Here's how the part is built. I have some questions about the finished solid (model axes, mm). Face numbers are marked on the shaded views. Round coordinates to 2 decimals unless told otherwise and drop trailing zeros. Write each loop counter-clockwise with the first axis right and the second up, starting at its lowest first coordinate (ties: lowest second). Pieces come first, ordered by that corner, then holes. Notation, with made-up numbers: M 44.5,18.25 L 77.5,18.25 A35 cw 77.5,57.25 Z; hole C 73.25,74.25 d3. An arc over 180 degrees is marked long. Write item = value, one per line. Start each with the question number.
(1) I want a section at D-D (x = 54). List the corners of the cut face in (y, z) for me.
(2) I want a section at A-A (z = -33). List the corners of the cut face in (x, y) for me.
(3) I need wall thicknesses on line 1 along X through (y, z) = (4, -66); line 2 along Y through (x, z) = (2.2, -33); line 3 along X through (y, z) = (7.5, -65). Which ranges of each line are inside material? Lowest first, please.
(4) If we mould it in two halves opening along Z, with no side actions, what happens to the marked faces 1, 2, 3 and 4? For each: released by +Z, released by -Z, zero draft, split by the parting line, or undercut.
(5) Will these pins go through, and if not, where does the flat tip stop? pin 1 Ø1 at (y, z) = (21, -61.5) entering from +X; pin 2 Ø0.6 at (x, y) = (50, 12.5) entering from +Z; pin 3 Ø0.8 at (x, z) = (78, -77.5) entering from +Y.
(6) I want a section at C-C (y = 5.5). Give the number of separate pieces and of enclosed holes in the cut face, and give its area (3 significant figures).
(7) I want a section at B-B (z = -54). List the corners of the cut face in (x, y) for me, and give its area (3 significant figures).
Autodesk Fusion 360 part; units mm, degrees
sketch "Sketch1" plane through (0, 0, 0) normal (0, 1, 0) x (1, 0, 0)
  line L0 (0, 0) -> (120, 0)
  line L1 (120, 0) -> (120, 85)
  line L2 (120, 85) -> (0, 85)
  line L3 (0, 85) -> (0, 0)
extrude "Extrude1" add sketch "Sketch1" along normal blind 3
sketch "Sketch2" plane through (0, 3, 0) normal (0, 1, 0) x (-1, 0, 0)
  line L0 (0, -85) -> (0, 0)
  line L1 (0, 0) -> (-120, 0)
  line L2 (-120, 0) -> (-120, -85)
  line L3 (-120, -85) -> (0, -85)
  line L4 (-60, -85) -> (-60, 0)
  line L5 (-60, -76.9514) -> (-120, -76.9514)
  line L6 (-77.8086, -80) -> (-77.8086, -73)
  circle A0 centre (-77.8086, -76.9514) radius 3.5
  circle A1 centre (-105.7039, -76.9514) radius 3.5
  dimension "d3" = 7
  dimension "d4" = 7
sketch "Sketch3" plane through (0, 3, 0) normal (0, 1, 0) x (-1, 0, 0)
  line L0 (-60, -10.9513) -> (-119.9962, -10.9513)
  line L1 (-60, -85) -> (-60, 0)
  line L2 (-60, -26.1629) -> (-72, -26.1629)
  line L3 (-62.566, -28.9848) -> (-62.566, -23)
  circle A0 centre (-62.566, -26.1629) radius 3.5
  line L4 (-107.0217, -24.9659) -> (-120.1868, -24.9659)
  line L5 (-110.7456, -28) -> (-110.7456, -22)
  circle A1 centre (-110.7456, -25) radius 2.5
  line L6 (-55, 0) -> (-55.9638, 0)
  line L7 (-55.9638, 0) -> (-55.9638, -85)
  line L8 (-55.9638, -85) -> (-55, -85)
  line L9 (-55, -85) -> (-55, 0)
  line L10 (0, 0) -> (-120, 0)
  line L11 (-120, -85) -> (0, -85)
  dimension "d5" = 7
  dimension "d6" = 5
extrude "Extrude2" add sketch "Sketch2" sketch "Sketch3" along normal blind 5 contours L5 A0 | L5 L6 A0 | L5 A1 | L5 A1 | L5 L6 A0 of sketch 2 contours L1 A0 | L1 L2 A0 | L1 L2 A0 | L4 L5 A1 | L4 L5 A1 | L4 L5 A1 | L4 L5 A1
hole "Hole1" at (77.8086, 8, -76.9514) direction (0, -1, 0) diameter 2.529 depth 4 tip angle 180
hole "Hole2" at (105.7039, 8, -76.9514) direction (0, -1, 0) diameter 2.529 depth 4 tip angle 180
hole "Hole3" at (62.566, 8, -26.1629) direction (0, -1, 0) diameter 2.529 depth 4 tip angle 180
hole "Hole4" at (110.7456, 8, -25) direction (0, -1, 0) diameter 2.529 depth 4 tip angle 180
sketch "Sketch4" plane through (0, 3, 0) normal (0, 1, 0) x (-1, 0, 0)
  circle A0 centre (-62.566, -26.1629) radius 3.5
  circle A1 centre (-105.7039, -76.9514) radius 3.5
  circle A2 centre (-77.8086, -76.9514) radius 3.5
  circle A3 centre (-110.7456, -25) radius 2.5
  line L0 (0, -85) -> (0, 0)
  line L1 (0, 0) -> (-120, 0)
  line L2 (-120, 0) -> (-120, -85)
  line L3 (-120, -85) -> (0, -85)
  line L4 (-50, -15) -> (-22, -15)
  line L5 (-22, -15) -> (-22, -70)
  line L6 (-22, -70) -> (-50, -70)
  line L7 (-50, -70) -> (-50, -15)
  line L8 (-22, -18) -> (-50, -18)
  circle A4 centre (-25, -18) radius 3
  circle A5 centre (-47, -18) radius 3
  line L9 (-20, -70) -> (-52, -70)
  line L10 (-52, -70) -> (-52, -69)
  line L11 (-52, -69) -> (-20, -69)
  line L12 (-20, -69) -> (-20, -70)
  dimension "d21" = 6
  dimension "d22" = 6
extrude "Extrude3" add sketch "Sketch4" along normal blind 5 contours L8 A5 | L8 A5 | L8 A4 | L5 L6 L7 L9 L11 | L7 L9 L10 L11 | L8 A4 | L5 L9 L11 L12
hole "Hole5" at (25, 8, -18) direction (0, -1, 0) diameter 2.529 depth 4 tip angle 180
hole "Hole6" at (47, 8, -18) direction (0, -1, 0) diameter 2.529 depth 4 tip angle 180
sketch "Sketch5" plane through (0, 3, 0) normal (0, 1, 0) x (-1, 0, 0)
  circle A0 centre (-47, -18) radius 3
  circle A1 centre (-25, -18) radius 3
  line L0 (-20, -69) -> (-20, -70)
  line L1 (-20, -70) -> (-52, -70)
  line L2 (-52, -70) -> (-52, -69)
  line L3 (-52, -69) -> (-20, -69)
  circle A2 centre (-62.566, -26.1629) radius 3.5
  circle A3 centre (-105.7039, -76.9514) radius 3.5
  circle A4 centre (-77.8086, -76.9514) radius 3.5
  circle A5 centre (-110.7456, -25) radius 2.5
  line L4 (0, -85) -> (0, 0)
  line L5 (0, 0) -> (-120, 0)
  line L6 (-120, 0) -> (-120, -85)
  line L7 (-120, -85) -> (0, -85)
  line L8 (-20, -70) -> (-52, -70)
  line L9 (-52, -70) -> (-52, -73)
  line L10 (-52, -73) -> (-20, -73)
  line L11 (-20, -73) -> (-20, -70)
extrude "Extrude4" add sketch "Sketch5" along normal blind 5 contours L1 L8 L9 L10 L11
sketch "Sketch6" plane through (0, 8, 0) normal (0, 1, 0) x (-1, 0, 0)
  line L0 (-20, -69) -> (-52, -69)
  line L1 (-52, -69) -> (-52, -73)
  line L2 (-52, -73) -> (-20, -73)
  line L3 (-20, -73) -> (-20, -69)
  line L4 (-20, -73) -> (-52, -73)
  line L5 (-52, -73) -> (-52, -71)
  line L6 (-52, -71) -> (-20, -71)
  line L7 (-20, -71) -> (-20, -73)
extrude "Extrude5" add sketch "Sketch6" along normal blind 5 contours L1 L2 L3 L4 L5 L6 L7
sketch "Sketch7" plane through (0, 0, -71) normal (0, 0, 1) x (1, 0, 0)
  line L0 (20, 8) -> (52, 8)
  line L1 (52, 8) -> (52, 13)
  line L2 (52, 13) -> (20, 13)
  line L3 (20, 13) -> (20, 8)
  line L4 (48.0761, 13) -> (52, 13)
  line L5 (52, 13) -> (52, 10.5)
  line L6 (52, 10.5) -> (48.0761, 10.5)
  line L7 (48.0761, 10.5) -> (48.0761, 13)
extrude "Extrude6" add sketch "Sketch7" along normal blind 4 contours L1 L2 L4 L5 L6 L7
sketch "Sketch8" plane through (52, 0, 0) normal (1, 0, 0) x (0, 0, -1)
  line L0 (69, 3) -> (73, 3)
  line L1 (73, 3) -> (73, 13)
  line L2 (73, 13) -> (67, 13)
  line L3 (67, 13) -> (67, 10.5)
  line L4 (67, 10.5) -> (71, 10.5)
  line L5 (71, 10.5) -> (71, 8)
  line L6 (71, 8) -> (69, 8)
  line L7 (69, 8) -> (69, 3)
  line L8 (67, 11.75) -> (71, 10.5)
extrude "Extrude7" cut sketch "Sketch8" against normal blind 4 contours L3 L4 L8
sketch "Sketch9" plane through (0, 3, 0) normal (0, 1, 0) x (-1, 0, 0)
  line L0 (-52, -73) -> (-52, -69)
  line L1 (-52, -69) -> (-20, -69)
  line L2 (-20, -69) -> (-20, -73)
  line L3 (-20, -73) -> (-52, -73)
  circle A0 centre (-47, -18) radius 3
  circle A1 centre (-25, -18) radius 3
  circle A2 centre (-62.566, -26.1629) radius 3.5
  circle A3 centre (-105.7039, -76.9514) radius 3.5
  circle A4 centre (-77.8086, -76.9514) radius 3.5
  circle A5 centre (-110.7456, -25) radius 2.5
  line L4 (0, -85) -> (0, 0)
  line L5 (0, 0) -> (-120, 0)
  line L6 (-120, 0) -> (-120, -85)
  line L7 (-120, -85) -> (0, -85)
  line L8 (0, 0) -> (-2.9371, 0)
  line L9 (-2.9371, 0) -> (-2.9371, -85)
  line L10 (-2.9371, -85) -> (0, -85)
  line L11 (0, -85) -> (0, 0)
  line L12 (0, 0) -> (-3, 0)
  line L13 (-3, 0) -> (-3, -85)
  line L14 (-3, -85) -> (0, -85)
  line L15 (0, -85) -> (0, 0)
  dimension "d39" = 3
extrude "Extrude8" add sketch "Sketch9" along normal blind 30 contours L4 L5 L7 L8 L9 L10 L11 L12 L14 L15
sketch "Sketch10" plane through (2.9371, 0, 0) normal (1, 0, 0) x (0, 0, -1)
  line L0 (0, 3) -> (85, 3)
  line L1 (85, 3) -> (85, 33)
  line L2 (85, 33) -> (0, 33)
  line L3 (0, 33) -> (0, 3)
  line L4 (0, 33) -> (3, 33)
  line L5 (3, 33) -> (3, 3)
  line L6 (3, 3) -> (0, 3)
  line L7 (0, 3) -> (0, 33)
  line L8 (85, 33) -> (82, 33)
  line L9 (82, 33) -> (82, 3)
  line L10 (82, 3) -> (85, 3)
  line L11 (85, 3) -> (85, 33)
  dimension "d42" = 3
  dimension "d43" = 3
extrude "Extrude9" add sketch "Sketch10" along normal blind 15 contours L0 L2 L3 L4 L5 L6 L7 | L0 L1 L2 L8 L9 L10 L11
sketch "Sketch11" plane through (0, 0, -3) normal (0, 0, -1) x (-1, 0, 0)
  line L0 (-2.9371, 3) -> (-2.9371, 33)
  line L1 (-2.9371, 33) -> (-17.9371, 33)
  line L2 (-17.9371, 33) -> (-17.9371, 3)
  line L3 (-17.9371, 3) -> (-2.9371, 3)
  line L4 (-2.9371, 33) -> (-17.9371, 3)
extrude "Extrude10" cut sketch "Sketch11" against normal blind 4 contours L1 L2 L4
sketch "Sketch13" plane through (0, 3, 0) normal (0, 1, 0) x (-1, 0, 0)
  line L0 (-17.9371, -82) -> (-2.9371, -82)
  line L1 (-2.9371, -82) -> (-2.9371, -3)
  line L2 (-2.9371, -3) -> (-17.9371, -3)
  line L3 (-17.9371, -3) -> (-17.9371, 0)
  line L4 (-17.9371, 0) -> (-120, 0)
  line L5 (-120, 0) -> (-120, -85)
  line L6 (-120, -85) -> (-17.9371, -85)
  line L7 (-52, -73) -> (-52, -69)
  line L8 (-52, -69) -> (-20, -69)
  line L9 (-20, -69) -> (-20, -73)
  line L10 (-20, -73) -> (-52, -73)
  circle A0 centre (-47, -18) radius 3
  circle A1 centre (-25, -18) radius 3
  circle A2 centre (-62.566, -26.1629) radius 3.5
  circle A3 centre (-105.7039, -76.9514) radius 3.5
  circle A4 centre (-77.8086, -76.9514) radius 3.5
  circle A5 centre (-110.7456, -25) radius 2.5
  line L11 (-14.9586, -82) -> (-17.7256, -82)
  line L12 (-17.7256, -82) -> (-17.7256, -39)
  line L13 (-17.7256, -39) -> (-14.9586, -39)
  line L14 (-14.9586, -39) -> (-14.9586, -82)
  line L15 (-17.9371, -85) -> (-17.9371, -82)
extrude "Extrude12" add sketch "Sketch13" along normal blind 25 contours L0 L11 L12 L13 L14
sketch "Sketch14" plane through (0, 0, -82) normal (0, 0, 1) x (1, 0, 0)
  line L0 (17.7256, 28) -> (17.7256, 3)
  line L1 (17.7256, 3) -> (17.9371, 3)
  line L2 (17.9371, 3) -> (17.9371, 33)
  line L3 (17.9371, 33) -> (2.9371, 33)
  line L4 (2.9371, 33) -> (2.9371, 3)
  line L5 (2.9371, 3) -> (14.9586, 3)
  line L6 (14.9586, 3) -> (14.9586, 28)
  line L7 (14.9586, 28) -> (17.7256, 28)
  line L8 (2.9371, 33) -> (14.9586, 28)
extrude "Extrude13" cut sketch "Sketch14" against normal blind 4 contours L0 L1 L2 L3 L7 L8
sketch "Sketch15" plane through (0, 0, 0) normal (-1, 0, 0) x (0, 0, 1)
  line L0 (-85, 0) -> (0, 0)
  line L1 (0, 0) -> (0, 33)
  line L2 (0, 33) -> (-85, 33)
  line L3 (-85, 33) -> (-85, 0)
  line L4 (-77, 8) -> (-43, 8)
  line L5 (-43, 8) -> (-43, 22.5)
  line L6 (-43, 22.5) -> (-77, 22.5)
  line L7 (-77, 22.5) -> (-77, 8)
  dimension "d54" = 34
  dimension "d55" = 14.5
extrude "Extrude14" cut sketch "Sketch15" against normal blind 5 contours L4 L5 L6 L7
sketch "Sketch16" plane through (0, 0, 0) normal (-1, 0, 0) x (0, 0, 1)
  line L0 (-43, 8) -> (-77, 8)
  line L1 (-77, 8) -> (-77, 22.5)
  line L2 (-77, 22.5) -> (-43, 22.5)
  line L3 (-43, 22.5) -> (-43, 8)
  line L4 (-85, 0) -> (0, 0)
  line L5 (0, 0) -> (0, 33)
  line L6 (0, 33) -> (-85, 33)
  line L7 (-85, 33) -> (-85, 0)
  circle A0 centre (-15, 15) radius 8
  circle A1 centre (-33, 25) radius 3.5
  dimension "d58" = 16
  dimension "d59" = 7
extrude "Extrude15" cut sketch "Sketch16" against normal blind 4 contours A0 | A1
fillet "Fillet1" radius 5 1 edges at (16.3421, 28, -39)
fillet "Fillet2" radius 1 4 edges at (1.4685, 33, 0) (10.4371, 18, 0) (10.4371, 18, -3) (0, 33, -42.5)
fillet "Fillet3" radius 1 3 edges at (17.7256, 13, -39) (17.7256, 26.5355, -40.4645) (17.7256, 28, -64.5)
sketch "Sketch17" plane through (0, 3, 0) normal (0, 1, 0) x (-1, 0, 0)
  circle A0 centre (-110.7456, -25) radius 2.5
  circle A1 centre (-77.8086, -76.9514) radius 3.5
  circle A2 centre (-105.7039, -76.9514) radius 3.5
  circle A3 centre (-62.566, -26.1629) radius 3.5
  circle A4 centre (-25, -18) radius 3
  circle A5 centre (-47, -18) radius 3
  line L0 (-52, -73) -> (-52, -69)
  line L1 (-52, -69) -> (-20, -69)
  line L2 (-20, -69) -> (-20, -73)
  line L3 (-20, -73) -> (-52, -73)
  line L4 (-16.7256, -39) -> (-14.9586, -39)
  line L5 (-14.9586, -39) -> (-14.9586, -82)
  line L6 (-14.9586, -82) -> (-2.9371, -82)
  line L7 (-2.9371, -82) -> (-2.9371, -3)
  line L8 (-2.9371, -3) -> (-16.8191, -3)
  ellipse E0 centre (-16.8191, -2) end of major axis (-17.9371, -2) minor radius 1 (-17.9371, -2) -> (-16.8191, -3) ccw
  line L9 (-17.9371, -2) -> (-17.9371, -1)
  ellipse E1 centre (-16.8191, -1) end of major axis (-17.9371, -1) minor radius 1 (-16.8191, 0) -> (-17.9371, -1) ccw
  line L10 (-16.8191, 0) -> (-120, 0)
  line L11 (-120, 0) -> (-120, -85)
  line L12 (-120, -85) -> (-17.7256, -85)
  line L13 (-17.7256, -85) -> (-17.7256, -40)
  arc A6 (-16.7256, -39) -> (-17.7256, -40) centre (-16.7256, -40) ccw
  line L14 (-8.6438, -82) -> (-7, -82)
  line L15 (-7, -82) -> (-7, -40)
  line L16 (-7, -40) -> (-8.6438, -40)
  line L17 (-8.6438, -40) -> (-8.6438, -82)
extrude "Extrude16" add sketch "Sketch17" along normal blind 4 contours L6 L14 L15 L16 L17
sketch "Sketch18" plane through (0, 0, -82) normal (0, 0, 1) x (1, 0, 0)
  line L0 (8.6438, 7) -> (8.6438, 3)
  line L1 (8.6438, 3) -> (14.9586, 3)
  line L2 (14.9586, 3) -> (14.9586, 28)
  line L3 (14.9586, 28) -> (2.9371, 33)
  line L4 (2.9371, 33) -> (2.9371, 3)
  line L5 (2.9371, 3) -> (7, 3)
  line L6 (7, 3) -> (7, 7)
  line L7 (7, 7) -> (8.6438, 7)
  line L8 (7, 7) -> (8.6319, 7)
  line L9 (8.6319, 7) -> (8.6319, 25.0515)
  line L10 (8.6319, 25.0515) -> (7, 25.0515)
  line L11 (7, 25.0515) -> (7, 7)
extrude "Extrude17" add sketch "Sketch18" along normal blind 3 contours L7 L8 L9 L10 L11
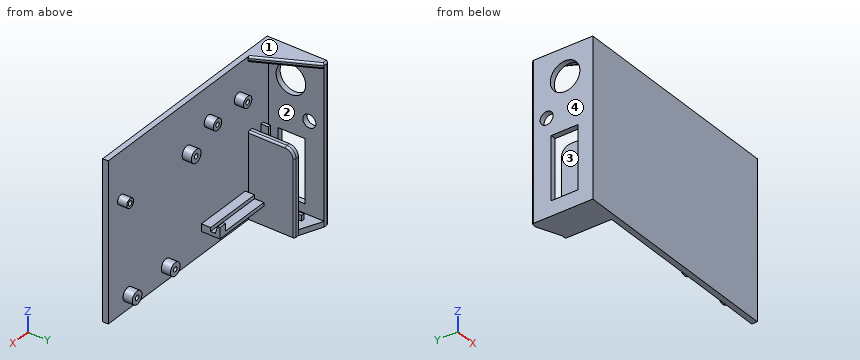
Returned:
q1.outline = M 0,-85 L 3,-85 L 3,0 L 0,0 Z
q2.outline = M 0,0 L 120,0 L 120,3 L 2.94,3 L 2.94,21.5 L 0,21.5 Z; M 0,28.5 L 2.94,28.5 L 2.94,33 L 1,33 A1 ccw 0,32 Z
q3.line_1 = 0 to 2.94, 7 to 8.64, 14.96 to 17.73
q3.line_2 = 0 to 21.5, 28.5 to 33
q3.line_3 = 0 to 2.94, 14.96 to 17.73
q4.face_1 = released by +Z
q4.face_2 = undercut
q4.face_3 = undercut
q4.face_4 = zero draft
q5.pin_1 = 17.73
q5.pin_2 = -67
q5.pin_3 = 4
q6.separate_pieces = 8
q6.enclosed_holes = 6
q6.area = 812 mm²
q7.outline = M 0,0 L 120,0 L 120,3 L 17.73,3 L 17.73,27 A1 ccw 16.73,28 L 14.96,28 L 14.96,3 L 8.64,3 L 8.64,7 L 7,7 L 7,3 L 2.94,3 L 2.94,8 L 0,8 Z; M 0,22.5 L 2.94,22.5 L 2.94,33 L 1,33 A1 ccw 0,32 Z
q7.area = 481 mm²
